from build123d import *

# Parameters (mm, degrees)
SKETCH1_W              = 15
SKETCH1_H              = 6
MAIN_BODY_DEPTH        = 5
SKETCH3_R              = 1.25
GRIN_HOLE_DEPTH        = 4
SKETCH2_R              = 0.795
MAGNET_HOLES_DEPTH     = 1
SET_SCREW_INDENT_DEPTH = 6


with BuildPart() as part:
    # Sketch1 → Main Body (new body)
    with BuildSketch(Plane(origin=(0, 0, 0), x_dir=(1, 0, 0), z_dir=(0, 1, 0))):
        Rectangle(SKETCH1_W, SKETCH1_H)
    extrude(amount=MAIN_BODY_DEPTH)

    # Sketch3 → GRIN Hole (cut)
    with BuildSketch(Plane.XZ):
        with Locations((-4.5, 0)):
            Circle(SKETCH3_R)
    extrude(amount=-GRIN_HOLE_DEPTH, mode=Mode.SUBTRACT)

    # Sketch2 → Magnet Holes (cut)
    with BuildSketch(Plane.XZ):
        with Locations((-6.25, -1.875)):
            Circle(SKETCH2_R)
        with Locations((-6.25, 1.875)):
            Circle(SKETCH2_R)
        with Locations((2.5, 0)):
            Circle(SKETCH2_R)
    extrude(amount=-MAGNET_HOLES_DEPTH, mode=Mode.SUBTRACT)

    # Sketch4 → Set Screw Indent (cut, through all)
    with BuildSketch(Plane.XZ):
        Polygon((7.058045095, -3), (7.5, -1.895112738), (7.5, -3), align=None)
    extrude(amount=-SET_SCREW_INDENT_DEPTH, mode=Mode.SUBTRACT)


solid = part.part
Could you check a few things on this model? Use its own coordinates, in mm. A direction names the side the tool comes from. Coordinates: 2 decimals unless noted, no trailing zeros. Loops run counter-clockwise (first coordinate to the right, second up) from the corner with the lowest first, then second, coordinate; pieces in that order, holes last.
1. I need wall thicknesses on L1, parallel to X at y = 3.2, z = 0.1; L2, parallel to Z at x = 2.5, y = 0.5 (3 decimals); L3, parallel to Z at x = -4.5, y = 1.65. Which ranges of each line are inside material? Lowest first, please.
2. Imagine slicing it at C-C (x = 2.5). Please give me the cut outline in (y, z) (3 decimals).
3. Imagine slicing it at A-A (z = 0). Please give me the cut outline in (x, y) (3 decimals), and give its area (3 significant figures).
4. We'd pull the mould along X, two halves only. Please class faces 3 (the face through (7.5, 2, 1)), 4 (the face through (0, 2, -3)), 5 (the face through (-6, 1, -2)): released by +X, released by -X, zero draft, split by the parting line, or undercut.
5. For faces 1 (the face through (0, 5, 0)), 2 (the face through (-6.88, 0.49, -2.36)), which set-ups out of +Z, -Z, +X, -X, +Y, -Y let a thin tool reach every point of the face, with its end or its side?
6. Imagine slicing it at D-D (y = 0.85). Please give me the cut outline in (x, z) (3 decimals), and give its area (3 significant figures).
7. Imagine slicing it at B-B (y = 1.9). Please give me the cut outline in (x, z), and give its area (3 significant figures).
8. For P1, Ø0.5, axis at x = 3, z = 0, coming from the -Y side; P2, Ø2, axis at x = -4.5, z = 0, coming from the -Y side; P3, Ø1.8, axis at x = 2.5, z = 0, coming from the -Y side, each with a flat end and sliding along its axis, tell me the tip position at first contact or that it passes through.
Computed values:
1. L1: x = -7.5 to -5.75, -3.25 to 7.5
1. L2: z = -3 to -0.795, 0.795 to 3
1. L3: z = -3 to -1.25, 1.25 to 3
2. outline: (0, -3) - (5, -3) - (5, 3) - (0, 3) - (0, 0.795) - (1, 0.795) - (1, -0.795) - (0, -0.795) - close
3. outline: (-7.5, 0) - (-5.75, 0) - (-5.75, 4) - (-3.25, 4) - (-3.25, 0) - (1.705, 0) - (1.705, 1) - (3.295, 1) - (3.295, 0) - (7.5, 0) - (7.5, 5) - (-7.5, 5) - close
3. area: 63.4 mm2
4. face 3: released by +X
4. face 4: zero draft
4. face 5: undercut
5. face 1: +Z, -Z, +X, -X, +Y
5. face 2: -Y
6. outline: (-7.5, -3) - (7.058, -3) - (7.5, -1.895) - (7.5, 3) - (-7.5, 3) - close; hole circle Ø1.59 at (-6.25, -1.875); hole circle Ø1.59 at (-6.25, 1.875); hole circle Ø2.5 at (-4.5, 0); hole circle Ø1.59 at (2.5, 0)
6. area: 78.9 mm2
7. outline: (-7.5, -3) - (7.06, -3) - (7.5, -1.9) - (7.5, 3) - (-7.5, 3) - close; hole circle Ø2.5 at (-4.5, 0)
7. area: 84.8 mm2
8. P1: stops at y = 1
8. P2: stops at y = 4
8. P3: stops at y = 0
